Could you check a few things on this drawing? It's one solid part, dimensions in mm from its lowest x, y, z. A direction names the side the tool comes from. Coordinates: 2 decimals unless noted, no trailing zeros. Order: outer loops, then holes, each group sorted by start corner. A loop starts at its lowest first (then second) coordinate and runs counter-clockwise, first axis right, second up. Notation, with made-up numbers: (35, 83.25) -> (44, 83.25) arc R28 ccw to (44, 121.25) -> close; hole circle Ø11 at (60.25, 50). An arc over 180 degrees is marked (long way). Answer as CSV lines item,"result".
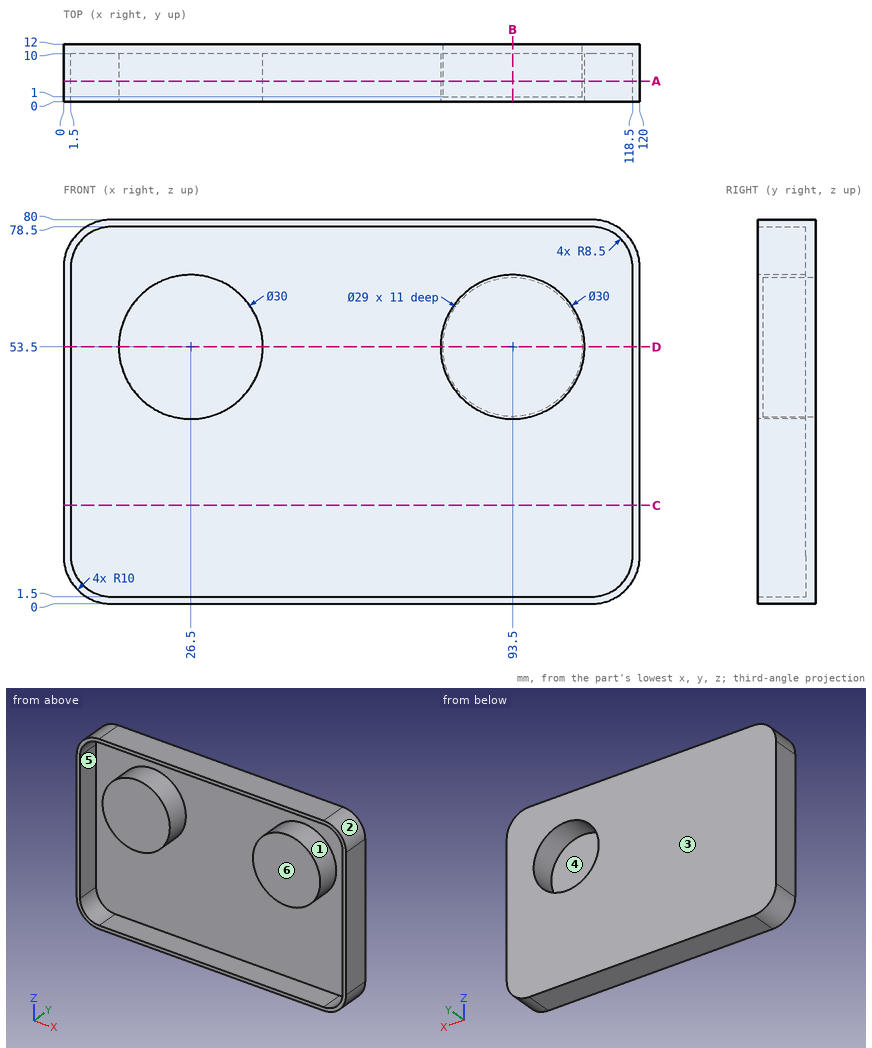
Q1. If I drill on line 1 (Z direction, x = 93.5, y = 9.75); line 2 (Z direction, x = 51.5, y = 7.5); line 3 (Z direction, x = 86.5, y = 5.5), over which ranges is the centre line in solid material (lowest first)?
Solution:
line 1,"0 to 1.5, 38.5 to 39, 68 to 68.5, 78.5 to 80"
line 2,"0 to 1.5, 78.5 to 80"
line 3,"0 to 1.5, 40.23 to 40.8, 66.2 to 66.77, 78.5 to 80"
Q2. Which directions (+Z, -Z, +X, -X, +Y, -Y) give clear straight access to the entire face, cutting with the end or side of a thin tool? Please do the marked faces 4, 5 and 6.
Solution:
face 4,"+Y"
face 5,"-Y"
face 6,"+Z, -Z, +X, -X, -Y"
Q3. Imagine slicing it at B-B (x = 93.5). List the corners of the cut face in (y, z) for me.
Solution:
outline,"(0, 0) -> (12, 0) -> (12, 39) -> (1, 39) -> (1, 68) -> (12, 68) -> (12, 80) -> (0, 80) -> (0, 78.5) -> (10, 78.5) -> (10, 68.5) -> (0, 68.5) -> (0, 38.5) -> (10, 38.5) -> (10, 1.5) -> (0, 1.5) -> close"
Q4. We'd pull the mould along X, two halves only. Please class the marked faces 1, 2 and 3: pulls with the +X half, pulls with the -X half, needs draft (parallel to the pull), parting line crosses it, or undercut.
Solution:
face 1,"undercut"
face 2,"pulls with the +X half"
face 3,"needs draft"
Q5. Imagine slicing it at D-D (z = 53.5). List the corners of the cut face in (x, y) for me, and give its area (3 significant figures).
Solution:
outline,"(0, 0) -> (1.5, 0) -> (1.5, 10) -> (11.5, 10) -> (11.5, 0) -> (41.5, 0) -> (41.5, 10) -> (78.5, 10) -> (78.5, 0) -> (108.5, 0) -> (108.5, 10) -> (118.5, 10) -> (118.5, 0) -> (120, 0) -> (120, 12) -> (108, 12) -> (108, 1) -> (79, 1) -> (79, 12) -> (0, 12) -> close"
area,"551 mm2"
Q6. Imagine slicing it at C-C (z = 20.5). List the corners of the cut face in (x, y) for me.
Solution:
outline,"(0, 0) -> (1.5, 0) -> (1.5, 10) -> (118.5, 10) -> (118.5, 0) -> (120, 0) -> (120, 12) -> (0, 12) -> close"
Q7. Imagine slicing it at A-A (y = 4.25). List the corners of the cut face in (x, z) for me, and give its area (3 significant figures).
Solution:
outline,"(0, 10) arc R10 ccw to (10, 0) -> (110, 0) arc R10 ccw to (120, 10) -> (120, 70) arc R10 ccw to (110, 80) -> (10, 80) arc R10 ccw to (0, 70) -> close; circle Ø30 at (26.5, 53.5); circle Ø30 at (93.5, 53.5); hole (1.5, 10) arc R8.5 ccw to (10, 1.5) -> (110, 1.5) arc R8.5 ccw to (118.5, 10) -> (118.5, 70) arc R8.5 ccw to (110, 78.5) -> (10, 78.5) arc R8.5 ccw to (1.5, 70) -> close; hole circle Ø29 at (93.5, 53.5)"
area,"1,320 mm2"
Q8. For P1, Ø17.5, axis at x = 93.5, z = 53.5, coming from the +Y side; P2, Ø1.5, axis at x = 13.5, z = 22.5, coming from the -Y side, each with a flat end and sliding along its axis, tell me the tip position at first contact or that it passes through.
Solution:
P1,"y = 1"
P2,"y = 10"
